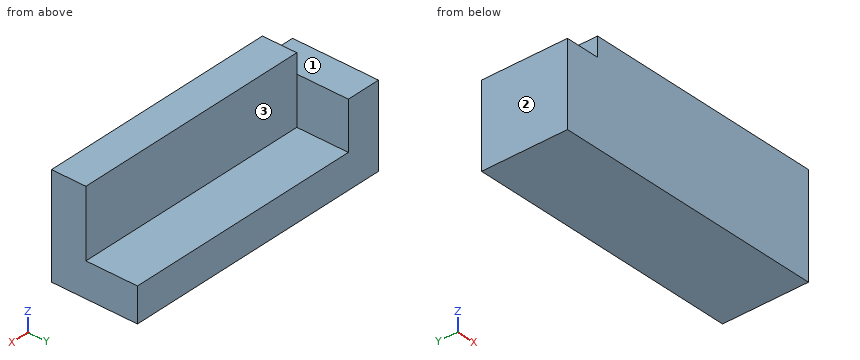
from build123d import *

# Parameters (mm, degrees)
F2_DEPTH = 3.175
F0_W     = 44.45
F0_H     = 6.35
F4_DEPTH = 6.35
F3_W     = 12.7
F3_H     = 15.24
F5_DEPTH = 6.35


with BuildPart() as f2:
    # F1 (on Front) → F2 (new body, symmetric)
    with BuildSketch(Plane.XZ):
        Polygon((0, 15.24), (0, 0), (50.8, 0), (50.8, 6.109729), (50.8, 18.809729), (6.35, 18.809729), (6.35, 15.24), align=None)
    extrude(amount=F2_DEPTH, both=True)

    # F0 (on Top) → F4 (join)
    with BuildSketch(Plane.XY):
        with Locations((28.575, 3.175)):
            Rectangle(F0_W, F0_H)
        Polygon((0, 0), (6.35, 0), (6.35, 6.35), (6.35, 12.7), (0, 12.7), align=None)
        with Locations((28.575, 9.525)):
            Rectangle(F0_W, F0_H)
    extrude(amount=F4_DEPTH)

    # F3 (on Right) → F5 (join)
    with BuildSketch(Plane.YZ):
        with Locations((6.35, 7.62)):
            Rectangle(F3_W, F3_H)
    extrude(amount=F5_DEPTH)


solid = f2.part
The model under review builds one solid part; all positions refer to its coordinate system, in mm. Face numbers are marked on the shaded views. A direction names the side the tool comes from. Round coordinates to 2 decimals unless told otherwise and drop trailing zeros. Order: outer loops, then holes, each group sorted by start corner. A loop starts at its lowest first (then second) coordinate and runs counter-clockwise, first axis right, second up. Notation, with made-up numbers: (65.5, 39) - (78.5, 39) arc R14 cw to (78.5, 57) - close; hole circle Ø9 at (-23, 88). An arc over 180 degrees is marked (long way). Use one line per item in the form item = value.
Q1. Add section A-A on y = -1.25. Give the boundary of the cut face in (x, z), then the cut area to 3 significant figures.
Response values:
outline = (0, 0) - (50.8, 0) - (50.8, 18.81) - (6.35, 18.81) - (6.35, 15.24) - (0, 15.24) - close
area = 933 mm^2
Q2. Clearance check with flat-ended pins moving along their axes: P1, Ø1.9, axis at x = 4, y = 6, coming from the +Z side; P2, Ø6, axis at x = 24.5, z = 11.5, coming from the +Y side (3 decimals); P3, Ø7, axis at y = 8.5, z = 12.5, coming from the +X side. State where each tip first meets the part, or that it passes through.
Response values:
P1 = 15.24
P2 = 3.175
P3 = 6.35
Q3. To check wall thickness, follow line 1 (Y direction, x = 35, z = 8) (3 decimals); line 2 (X direction, y = 9.75, z = 13.75). State the ranges of each line that lie inside material, in increasing order.
Response values:
line_1 = -3.175 to 3.175
line_2 = 0 to 6.35
Q4. Tool access review of the marked faces 1, 2 and 3: name each direction out of +Z, -Z, +X, -X, +Y, -Y from which nothing blocks a thin tool from reaching the whole face with its end or side.
Response values:
face_1 = +Z, -X, +Y, -Y
face_2 = +Z, -Z, -X, +Y, -Y
face_3 = +Z, +X, +Y
Q5. Add section B-B on z = 11.5. Give the boundary of the cut face in (x, y) (3 decimals), then the cut area to 3 significant figures.
Response values:
outline = (0, -3.175) - (50.8, -3.175) - (50.8, 3.175) - (6.35, 3.175) - (6.35, 12.7) - (0, 12.7) - close
area = 383 mm^2
Q6. Add section C-C on x = 4.5. Give the boundary of the cut face in (y, z) (3 decimals).
Response values:
outline = (-3.175, 0) - (12.7, 0) - (12.7, 15.24) - (-3.175, 15.24) - close
